Could you check a few things on this model? Use its own coordinates, in mm. A direction names the side the tool comes from. Round coordinates to 2 decimals unless told otherwise and drop trailing zeros. Write each loop counter-clockwise with the first axis right and the second up, starting at its lowest first coordinate (ties: lowest second). Pieces come first, ordered by that corner, then holes. Notation, with made-up numbers: (-13, 37) - (-6, 37) arc R16 cw to (-6, 45) - close; hole circle Ø10 at (76.5, 44.25). An arc over 180 degrees is marked (long way). Put each result on its own line as item: value.
from build123d import *

# Parameters (mm, degrees)
POCKET_DEPTH       = 418.517162
POLARPATTERN_COUNT = 5


with BuildPart() as part:
    # Sketch → Revolution (revolve)
    with BuildSketch(Plane.XZ):
        with BuildLine():
            ThreePointArc((45, 0), (52.071068, 2.928932), (55, 10))
            Line((55, 10), (55, 93))
            ThreePointArc((55, 93), (54.707107, 93.707107), (54, 94))
            Line((54, 94), (52, 94))
            Line((52, 94), (50, 92))
            Line((50, 92), (50, 89))
            Line((50, 89), (52, 87))
            Line((52, 87), (52, 10))
            ThreePointArc((45, 3), (49.949747, 5.050253), (52, 10))
            Line((20, 3), (45, 3))
            Line((20, 0), (20, 3))
            Line((45, 0), (20, 0))
        make_face()
    revolve(axis=Axis((0, 0, 0), (0, 0, 1)))

    # Sketch001 → Pocket (cut, through all)
    with BuildSketch(Plane.XZ):
        with BuildLine():
            ThreePointArc((-7.5, 35), (0, 27.5), (7.5, 35))
            Line((7.5, 35), (7.5, 159.742664))
            ThreePointArc((7.5, 159.742664), (0, 167.242664), (-7.5, 159.742664))
            Line((-7.5, 35), (-7.5, 159.742664))
        make_face()
    pocket = extrude(amount=-POCKET_DEPTH, mode=Mode.SUBTRACT)

    # PolarPattern: Pocket ×5 about axis
    polarpattern_axis = Axis((0, 0, 0), (0, 0, 1))
    for i in range(1, POLARPATTERN_COUNT):
        add(pocket.rotate(polarpattern_axis, i * 360 / POLARPATTERN_COUNT), mode=Mode.SUBTRACT)


solid = part.part
(1) Please list where these lines run through material, in increasing order: probe 1 along Y at (x, z) = (0, 1); probe 2 along X at (y, z) = (0, 58); probe 3 along Y at (x, z) = (0, 53). Write a range as from..to.
Values found:
probe 1: y = -49.36..-20, 20..49.36
probe 2: x = -55..-52, 52..55
probe 3: y = -55..-52
(2) I'm going to push flat-ended pins straight in: pin 1 (4 mm diameter, centred on y = 20, z = 24, fed in from -X); pin 2 (3 mm diameter, centred on y = 25, z = 46.5, fed in from +X); pin 3 (4 mm diameter, centred on y = -5, z = 30.5, fed in from +X). Where does each tip first touch, or does it pass through?
Values found:
pin 1: stops at x = -51.97
pin 2: stops at x = 49.5
pin 3: stops at x = 54.92
(3) Imagine slicing it at D-D, the plane z = 13.5. List the corners of the cut face in (x, y) for me, then the cut area to 3 significant figures.
Values found:
outline: circle Ø110 at (0, 0); hole circle Ø104 at (0, 0)
area: 1,010 mm^2
(4) Imagine slicing it at A-A, the plane x = 0. List the corners of the cut face in (y, z) for me, then the cut area to 3 significant figures.
Values found:
outline: (-55, 10) arc R10 ccw to (-45, 0) - (-20, 0) - (-20, 3) - (-45, 3) arc R7 cw to (-52, 10) - (-52, 87) - (-50, 89) - (-50, 92) - (-52, 94) - (-54, 94) arc R1 ccw to (-55, 93) - close; (20, 0) - (45, 0) arc R10 ccw to (55, 10) - (55, 27.5) - (52, 27.5) - (52, 10) arc R7 cw to (45, 3) - (20, 3) - close
area: 544 mm^2
(5) Imagine slicing it at C-C, the plane z = 82.5. List the corners of the cut face in (x, y) for me.
Values found:
outline: (-54.14, 9.7) arc R55 ccw to (-38.09, -39.67) - (-36.31, -37.22) arc R52 cw to (-51.26, 8.77) - close; (-49.5, 23.97) - (-46.62, 23.03) arc R52 cw to (-7.5, 51.46) - (-7.5, 54.49) arc R55 ccw to start; (-25.96, -48.49) arc R55 ccw to (25.96, -48.49) - (24.18, -46.04) arc R52 cw to (-24.18, -46.04) - close; (7.5, 51.46) arc R52 cw to (46.62, 23.03) - (49.5, 23.97) arc R55 ccw to (7.5, 54.49) - close; (36.31, -37.22) - (38.09, -39.67) arc R55 ccw to (54.14, 9.7) - (51.26, 8.77) arc R52 cw to start
(6) For faces 1 (the face through (-0.16, 53.2, 27.5)), 2 (the face through (48.134, 23.526, 64.087)), 3 (the face through (47.75, -15.87, 92.32)), which set-ups out of +Z, -Z, +X, -X, +Y, -Y let a thin tool reach every point of the face, with its end or its side?
Values found:
face 1: +Z, +Y
face 2: +Z, +X
face 3: +Z
(7) If we mould it in two halves opening along Z, with no side actions, what happens to faces 4 (the face through (-0.1, -52.4, 94)), 5 (the face through (-41.265, -31.641, 47.961)), 6 (the face through (0, -50, 90))? For each: pulls with the +Z half, pulls with the -Z half, needs draft (parallel to the pull), parting line crosses it, or undercut.
Values found:
face 4: pulls with the +Z half
face 5: undercut
face 6: needs draft
(8) Imagine slicing it at B-B, the plane y = 0. List the corners of the cut face in (x, z) for me.
Values found:
outline: (-55, 10) arc R10 ccw to (-45, 0) - (-20, 0) - (-20, 3) - (-45, 3) arc R7 cw to (-52, 10) - (-52, 87) - (-50, 89) - (-50, 92) - (-52, 94) - (-54, 94) arc R1 ccw to (-55, 93) - close; (20, 0) - (45, 0) arc R10 ccw to (55, 10) - (55, 93) arc R1 ccw to (54, 94) - (52, 94) - (50, 92) - (50, 89) - (52, 87) - (52, 10) arc R7 cw to (45, 3) - (20, 3) - close
